Verification items for the finished model (mm, model axes). Face numbers are marked on the shaded views. A direction names the side the tool comes from. Give positions to 0.01 mm unless a question says otherwise; leave off trailing zeros. Answer as CSV lines item,"result". Start each with the question number.
1) Tool access check on the marked faces 4, 5 and 6. Record the directions out of +Z, -Z, +X, -X, +Y, -Y that give a thin tool (end or side, any length) a straight path to the whole face; none if there is none.
2) Mould release check, pull along X, two halves, no side actions. Record for the marked faces 1, 2 and 3: released by +X, released by -X, zero draft, split by the parting line, or undercut.
3) Gauge pin test, flat ends, axial feed: pin 1 Ø4.5 at (x, z) = (-15.56, 15.56) entering from +Y; pin 2 Ø5.5 at (x, z) = (15.56, 15.56) entering from -Y; pin 3 Ø1 at (y, z) = (0, -7) entering from -X; pin 4 Ø5 at (x, z) = (0, 0) entering from -Y. Record the tip position at first contact, or that the pin passes through.
4) Sectioned sample at A-A on y = 0.75. Give the number of separate pieces and of enclosed holes in the cut face, and give its area (3 significant figures).
5) Material ranges on L1, parallel to X at y = 1, z = 15; L2, parallel to Y at x = 5, z = -10.5, recorded low to high.
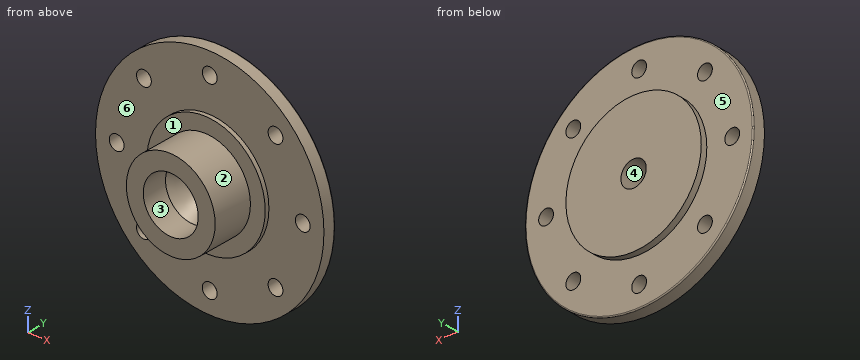
Autodesk Inventor part; units mm, degrees
ref_plane "YZ Plane" through (0, 0, 0) normal (1, 0, 0) x (0, 1, 0)
ref_plane "XZ Plane" through (0, 0, 0) normal (0, 1, 0) x (-1, 0, 0)
ref_plane "XY Plane" through (0, 0, 0) normal (0, 0, 1) x (1, 0, 0)
sketch "Sketch1" plane through (0, 0, 0) normal (0, 1, 0) x (-1, 0, 0)
  circle A0 centre (0, 0) radius 27
  dimension "d0" = 54
extrude "Extrusion1" add sketch "Sketch1" along normal blind 3
sketch "Sketch2" plane through (0, 3, 0) normal (0, 1, 0) x (1, 0, 0)
  circle A0 centre (0, 0) radius 16
  dimension "d4" = 32
extrude "Extrusion2" add sketch "Sketch2" along normal blind 1.5
sketch "Sketch3" plane through (0, 0, 0) normal (0, -1, 0) x (1, 0, 0)
  circle A0 centre (0, 0) radius 14
  dimension "d7" = 28
extrude "Extrusion3" add sketch "Sketch3" along normal blind 1
sketch "Sketch4" plane through (0, -1, 0) normal (0, -1, 0) x (1, 0, 0)
  circle A0 centre (0, 0) radius 10.5
  dimension "d10" = 21
extrude "Extrusion4" add sketch "Sketch4" along normal blind 9.5
sketch "Sketch6" plane through (0, 4.5, 0) normal (0, 1, 0) x (1, 0, 0)
  circle A0 centre (0, 0) radius 3
  dimension "d14" = 6
extrude "Extrusion5" cut sketch "Sketch6" against normal through all
sketch "Sketch7" plane through (0, 3, 0) normal (0, 1, 0) x (1, 0, 0)
  circle A0 centre (0, 0) radius 22 construction
  circle A1 centre (0, 22) radius 1.75
  circle A2 centre (-15.5563, 15.5563) radius 1.75
  circle A3 centre (-22, 0) radius 1.75
  circle A4 centre (-15.5563, -15.5563) radius 1.75
  circle A5 centre (0, -22) radius 1.75
  circle A6 centre (15.5563, -15.5563) radius 1.75
  circle A7 centre (22, 0) radius 1.75
  circle A8 centre (15.5563, 15.5563) radius 1.75
  dimension "d17" = 44
  dimension "d18" = 3.5
  dimension "d21" = 360
  dimension "d23" = 6.4436
extrude "Extrusion6" cut sketch "Sketch7" against normal blind 3
sketch "Sketch9" plane through (0, -10.5, 0) normal (0, -1, 0) x (1, 0, 0)
  circle A0 centre (0, 0) radius 6.5
  dimension "d26" = 13
extrude "Extrusion7" cut sketch "Sketch9" against normal blind 9.5
chamfer "Chamfer1" distance 3.5 angle 45 1 edges at (-6.5, -1, 0)
fillet "Fillet1" radius 0.25 1 edges at (27, 3, 0)
properties part number "Lower Cylinder Cover" material "Brass, Soft Yellow"
Ans:
1,face 4,"+Y, -Y"
1,face 5,"+Y"
1,face 6,"-Y"
2,face 1,"zero draft"
2,face 2,"split by the parting line"
2,face 3,"undercut"
3,pin 1,"stops at y = 3"
3,pin 2,"stops at y = 0"
3,pin 3,"stops at x = -26.21"
3,pin 4,"passes through"
4,separate pieces,"1"
4,enclosed holes,"9"
4,area,"2,180 mm²"
5,L1,"x = -22.45 to -17.22, -13.9 to 13.9, 17.22 to 22.45"
5,L2,"y = -1 to 4.5"
